Geometry: final body of the model. Coordinates: model frame, mm. Round coordinates to 2 decimals unless told otherwise and drop trailing zeros. Order: outer loops, then holes, each group sorted by start corner. A loop starts at its lowest first (then second) coordinate and runs counter-clockwise, first axis right, second up. Notation, with made-up numbers: (67.25, 40.5) -> (106.25, 40.5) arc R12 ccw to (106.25, 44.5) -> close; hole circle Ø3 at (10, -35.75). An arc over 180 degrees is marked (long way). Put each result on its own line as item: value.
```python
from build123d import *

# Parameters (mm, degrees)
SKETCH1_W          = 180
SKETCH1_H          = 165
BASE_FLANGE1_DEPTH = 3.175
FILLET1_R          = 10
SKETCH2_R          = 2.65
CUT_EXTRUDE1_DEPTH = 123.132430685
SKETCH3_R          = 2.65
CUT_EXTRUDE2_DEPTH = 123.132430685


# Sheet-metal steps are written as plain solids
with BuildPart() as part:
    # Sketch1 → Base-Flange1 (new body)
    with BuildSketch(Plane(origin=(0, 0, 0), x_dir=(1, 0, 0), z_dir=(0, 1, 0))):
        Rectangle(SKETCH1_W, SKETCH1_H)
    extrude(amount=-BASE_FLANGE1_DEPTH)

    # Fillet1
    fillet1_edges = [part.edges().sort_by_distance(p)[0] for p in [
        (90, -1.5875, 82.5),
        (-90, -1.5875, 82.5),
        (-90, -1.5875, -82.5),
        (90, -1.5875, -82.5),
    ]]
    fillet(fillet1_edges, radius=FILLET1_R)

    # Sketch2 → Cut-Extrude1 (cut, through all)
    with BuildSketch(Plane(origin=(0, 0, 0), x_dir=(1, 0, 0), z_dir=(0, 1, 0))):
        with Locations(Location((-80, 72.5, 0), (0, 0, 270))):
            Circle(SKETCH2_R)
        with Locations(Location((80, 72.5, 0), (0, 0, 270))):
            Circle(SKETCH2_R)
        with Locations(Location((-80, -72.5, 0), (0, 0, 270))):
            Circle(SKETCH2_R)
        with Locations(Location((80, -72.5, 0), (0, 0, 270))):
            Circle(SKETCH2_R)
    extrude(amount=-CUT_EXTRUDE1_DEPTH, mode=Mode.SUBTRACT)

    # Sketch3 → Cut-Extrude2 (cut, through all)
    with BuildSketch(Plane(origin=(0, 0, 0), x_dir=(1, 0, 0), z_dir=(0, 1, 0))):
        with Locations(Location((-79.8175, 52.1, 0), (0, 0, 270))):
            Circle(SKETCH3_R)
        with Locations(Location((-79.8175, 12.1, 0), (0, 0, 270))):
            Circle(SKETCH3_R)
        with BuildLine():
            Line((-20.41125, 54.35), (-14.41125, 54.35))
            ThreePointArc((-14.41125, 54.35), (-11.76125, 51.7), (-14.41125, 49.05))
            Line((-14.41125, 49.05), (-20.41125, 49.05))
            ThreePointArc((-20.41125, 49.05), (-23.06125, 51.7), (-20.41125, 54.35))
        make_face()
        with BuildLine():
            Line((-20.41125, 14.35), (-14.41125, 14.35))
            ThreePointArc((-14.41125, 14.35), (-11.76125, 11.7), (-14.41125, 9.05))
            Line((-14.41125, 9.05), (-20.41125, 9.05))
            ThreePointArc((-20.41125, 9.05), (-23.06125, 11.7), (-20.41125, 14.35))
        make_face()
    extrude(amount=-CUT_EXTRUDE2_DEPTH, mode=Mode.SUBTRACT)


solid = part.part
```
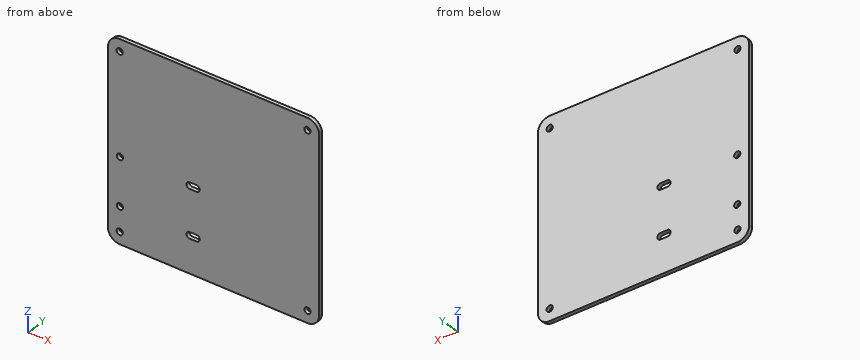
1. Contact query for a flat-ended pin moving along its axis: P1, Ø1, axis at x = -3.5, z = -24, coming from the +Y side. Output: stop coordinate, or through.
Ans:
P1: y = 0
2. Material intervals for probe 1 along X at (y, z) = (-1, -73); probe 2 along X at (y, z) = (-1.3, -52.1), sorted ascending.
Ans:
probe 1: -89.99 to -82.6, -77.4 to 77.4, 82.6 to 89.99
probe 2: -90 to -82.47, -77.17 to -23.03, -11.79 to 90
3. Cut plane A-A on z = -12.1. Return loops of the section in (x, y) (1 decimal), and give its area (3 significant figures).
Ans:
outline: (-90, -3.2) -> (-82.5, -3.2) -> (-82.5, 0) -> (-90, 0) -> close; (-77.2, -3.2) -> (-23, -3.2) -> (-23, 0) -> (-77.2, 0) -> close; (-11.8, -3.2) -> (90, -3.2) -> (90, 0) -> (-11.8, 0) -> close
area: 519 mm²
